```python
from build123d import *

# Parameters (mm, degrees)
BOSS_EXTRUDE1_DEPTH = 3
SKETCH2_R           = 2
BOSS_EXTRUDE2_DEPTH = 9
FILLET1_R           = 1.5
FILLET2_R           = 3
SKETCH3_R           = 2.5
CUT_EXTRUDE1_DEPTH  = 34.678628238


with BuildPart() as part:
    # Sketch1 → Boss-Extrude1 (new body)
    with BuildSketch(Plane(origin=(0, 0, 0), x_dir=(1, 0, 0), z_dir=(0, 1, 0))):
        Polygon((-15, 9), (-4.5, 23), (4.5, 23), (15, 9), (15, -9), (-15, -9), align=None)
    extrude(amount=BOSS_EXTRUDE1_DEPTH)

    # Sketch2 → Boss-Extrude2 (add)
    with BuildSketch(Plane(origin=(0, 0, -23), x_dir=(-1, 0, 0), z_dir=(0, 0, -1))):
        with BuildLine():
            Line((-4.5, 3), (-4.5, 18))
            ThreePointArc((-4.5, 18), (0, 22.5), (4.5, 18))
            Line((4.5, 18), (4.5, 3))
            Line((4.5, 3), (-4.5, 3))
        make_face()
        with Locations((0, 18)):
            Circle(SKETCH2_R, mode=Mode.SUBTRACT)
    extrude(amount=-BOSS_EXTRUDE2_DEPTH)

    # Fillet1
    fillet1_edges = [part.edges().sort_by_distance(p)[0] for p in [
        (0, 3, -14),
        (-4.5, 3, -18.5),
        (4.5, 3, -18.5),
    ]]
    fillet(fillet1_edges, radius=FILLET1_R)

    # Fillet2
    fillet2_edges = [part.edges().sort_by_distance(p)[0] for p in [
        (-15, 1.5, -9),
        (15, 1.5, -9),
        (15, 1.5, 9),
        (-15, 1.5, 9),
    ]]
    fillet(fillet2_edges, radius=FILLET2_R)

    # Sketch3 → Cut-Extrude1 (cut, through all)
    with BuildSketch(Plane(origin=(0, 3, 0), x_dir=(1, 0, 0), z_dir=(0, 1, 0))):
        with Locations(Location((-9, 0, 0), (0, 0, 270))):
            Circle(SKETCH3_R)
        with Locations(Location((9, 0, 0), (0, 0, 90))):
            Circle(SKETCH3_R)
    extrude(amount=-CUT_EXTRUDE1_DEPTH, mode=Mode.SUBTRACT)


solid = part.part
```
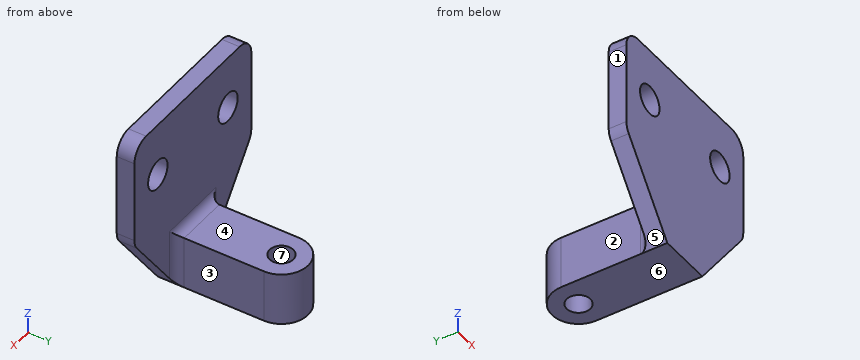
Design review of the part built by this model. Coordinates are the model's own, in mm. Face numbers are marked on the shaded views. A direction names the side the tool comes from. Coordinates: 2 decimals unless noted, no trailing zeros. Loops run counter-clockwise (first coordinate to the right, second up) from the corner with the lowest first, then second, coordinate; pieces in that order, holes last. Notation, with made-up numbers: (-3, 31) - (17, 31) arc R19 cw to (17, 38) - close; hole circle Ø11 at (-27.5, 82.5). An arc over 180 degrees is marked (long way). Use CSV: the item, a comma, the result in double quotes. Start each with the question number.
1) Consider section C-C on x = 0. Write out the cut boundary in (y, z).
2) Consider section D-D on y = 13. Write out the cut boundary in (x, z).
3) Tool access review of the marked faces 1, 2, 3 and 4: name each direction out of +Z, -Z, +X, -X, +Y, -Y from which nothing blocks a thin tool from reaching the whole face with its end or side.
4) For pin 1 Ø2 at (x, z) = (10, -6) entering from +Y; pin 2 Ø2.5 at (y, z) = (11, -16.5) entering from -X; pin 3 Ø3 at (x, y) = (0, 18) entering from +Z; pin 4 Ø4.5 at (y, z) = (13.5, -19.5) entering from +X, all flat-tipped, find the tip position at first contact; note any pin that passes through.
5) The part is to be moulded in two halves that separate along X. For the marked faces 5, 6 and 7, say which applies: +X half, -X half, draft (parallel to the pull), parting line (faces both ways), or undercut.
6) Wall thickness on L1, parallel to X at y = 1.9, z = 0; L2, parallel to Y at x = 6, z = -15; L3, parallel to X at y = 11.5, z = -15: over which ranges is each line inside the solid? List them lowest first. Write a range as from..to.
7) Consider section A-A on x = -9. Write out the cut boundary in (y, z).
8) Consider section B-B on z = 0. Write out the cut boundary in (x, y), then the cut area to 3 significant figures.
Geometry says:
1,outline,"(0, -23) - (16, -23) - (16, -14) - (4.5, -14) arc R1.5 cw to (3, -12.5) - (3, 9) - (0, 9) - close; (20, -23) - (22.5, -23) - (22.5, -14) - (20, -14) - close"
2,outline,"(-4.5, -23) - (4.5, -23) - (4.5, -14) - (-4.5, -14) - close"
3,face 1,"+Z, -Z, -X, +Y, -Y"
3,face 2,"+Z, -Z, -X, +Y"
3,face 3,"+Z, -Z, +X, +Y"
3,face 4,"+Z, +X, -X, +Y"
4,pin 1,"y = 3"
4,pin 2,"x = -4.5"
4,pin 3,"through"
4,pin 4,"x = 4.5"
5,face 5,"-X half"
5,face 6,"draft"
5,face 7,"undercut"
6,L1,"-15..-11.5, -6.5..6.5, 11.5..15"
6,L2,"0..3"
6,L3,"-4.5..4.5"
7,outline,"(0, -17) - (3, -17) - (3, -2.5) - (0, -2.5) - close; (0, 2.5) - (3, 2.5) - (3, 9) - (0, 9) - close"
8,outline,"(-15, 0) - (-11.5, 0) - (-11.5, 3) - (-15, 3) - close; (-6.5, 0) - (6.5, 0) - (6.5, 3) - (-6.5, 3) - close; (11.5, 0) - (15, 0) - (15, 3) - (11.5, 3) - close"
8,area,"60.0 mm^2"
